Verification items for the finished model (mm, model axes). A direction names the side the tool comes from. Give positions to 0.01 mm unless a question says otherwise; leave off trailing zeros. Loops run counter-clockwise (first coordinate to the right, second up) from the corner with the lowest first, then second, coordinate; pieces in that order, holes last. Notation, with made-up numbers: (68, 18) - (93, 18) arc R11 ccw to (93, 34) - close; hole circle Ø1 at (53, 72.25). An arc over 180 degrees is marked (long way). Use one line per item in the form item = value.
Autodesk Inventor part; units mm, degrees
ref_plane "YZ Plane" through (0, 0, 0) normal (1, 0, 0) x (0, 1, 0)
ref_plane "XZ Plane" through (0, 0, 0) normal (0, 1, 0) x (-1, 0, 0)
ref_plane "XY Plane" through (0, 0, 0) normal (0, 0, 1) x (1, 0, 0)
sketch "Sketch1" plane through (0, 0, 0) normal (0, 0, 1) x (1, 0, 0)
  line L0 (0, 0) -> (0, 125)
  line L1 (0, 125) -> (-105, 10)
  line L2 (-105, 10) -> (-105, 0)
  line L3 (-105, 0) -> (0, 0)
  line L4 (-100, 8.0608) -> (-5, 112.1084)
  line L5 (-5, 112.1084) -> (-5, 5)
  line L6 (-5, 5) -> (-100, 5)
  line L7 (-100, 5) -> (-100, 8.0608)
  point P0 (-52.5, 62.5)
  point P1 (-52.5, 0)
  point P2 (0, 62.5)
  dimension "d0" = 10
  dimension "d1" = 105
  dimension "d2" = 125
  dimension "d3" = 5
extrude "Extrusion1" add sketch "Sketch1" along normal blind 20
sketch "Sketch2" plane through (0, 0, 0) normal (0, 0, -1) x (-1, 0, 0)
  line L0 (5, 112.1084) -> (5, 5)
  line L1 (5, 8.8556) -> (50.4993, 62.2758)
  line L2 (100, 8.0608) -> (5, 112.1084)
  line L3 (5, 5) -> (100, 5)
  line L4 (8.2839, 5) -> (53.8973, 58.5542)
  line L5 (16.4791, 22.3331) -> (16.4791, 99.536)
  line L6 (21.4791, 94.0598) -> (21.4791, 28.2035)
  line L7 (24.1213, 23.5946) -> (85.817, 23.5946)
  line L8 (19.8627, 18.5946) -> (90.3822, 18.5946)
  line L9 (100, 5) -> (100, 8.0608)
  line L10 (100, 6.5304) -> (23.4466, 22.8023)
  line L11 (83.1512, 5) -> (19.7602, 18.4742)
  line L12 (8.1824, 108.6229) -> (21.0073, 27.6496)
  line L13 (5, 96.7537) -> (16.7388, 22.6379)
  point P0 (0, 0)
  point P1 (16.4791, 56.2397)
  point P2 (43.2425, 18.5946)
  point P3 (16.4791, 24.2774)
  dimension "d8" = 2.5
  dimension "d9" = 2.5
  dimension "d10" = 5
  dimension "d11" = 5
  dimension "d16" = 5
  dimension "d17" = 12
  dimension "d18" = 5
  dimension "d19" = 9
extrude "Extrusion2" add sketch "Sketch2" against normal blind 20 contours L2 L12 L5 L13 L0 | L1 L2 L4 L3 L0 | L13 L1 L5 | L5 L12 L1 L13 | L2 L6 L1 L12 L5 | L11 L4 L8 L10 L9 L3 | L4 L10 L8 | L2 L8 L10 L4 L7
fillet "Fillet1" radius 3 18 edges at (-90.3822, 18.5946, 10) (-53.8973, 58.5542, 10) (-85.817, 23.5946, 10) (-24.1213, 23.5946, 10) (-50.4993, 62.2758, 10) (-21.4791, 94.0598, 10) (-16.4791, 99.536, 10) (-21.4791, 28.2035, 10) (0, 0, 10) (-5, 8.8556, 10) (-8.2839, 5, 10) (-105, 0, 10) (-100, 8.0608, 10) (-105, 10, 10) (0, 125, 10) (-19.7602, 18.4742, 10) (-100, 6.5304, 10) (-8.1824, 108.6229, 10)
fillet "Fillet2" radius 1.5 4 edges at (-16.4791, 56.2397, 10) (-43.2425, 18.5946, 10) (-5, 96.7537, 10) (-83.1512, 5, 10)
sketch "Sketch5" plane through (0, 0, 20) normal (0, 0, 1) x (1, 0, 0)
  line L0 (-102, 0) -> (-3, 0)
  line L1 (-85, 0) -> (-85, -20)
  line L2 (-80, 0) -> (-80, -20)
  line L3 (-80, -20) -> (-85, -20)
  line L4 (-10, 0) -> (-10, -20)
  line L5 (-10, -20) -> (-5, -20)
  line L6 (-5, -20) -> (-5, 0)
  line L7 (-105, 8.8365) -> (-105, 3)
  point P0 (0, 0)
  dimension "d35" = 5
  dimension "d36" = 20
  dimension "d37" = 80
  dimension "d38" = 5
  dimension "d52" = 20
extrude "Extrusion3" add sketch "Sketch5" against normal up to surface (20 mm away)
fillet "Fillet3" radius 1.5 4 edges at (-80, -20, 10) (-85, -20, 10) (-10, -20, 10) (-5, -20, 10)
fillet "Fillet4" radius 10 2 edges at (-80, 0, 10) (-10, 0, 10)
sketch "Sketch6" plane through (-10, -18.5, 0) normal (-1, 0, 0) x (0, 0, 1)
  line L0 (0, -1.5) -> (20, -1.5)
  line L1 (0, 0) -> (0, 8.5)
  point P0 (0, 18.5)
  point P1 (10, 8.5)
  dimension "d50" = 10
  dimension "d51" = 10
hole "Hole2" at (-10, -10, 10) direction (1, 0, 0) diameter 5.8 end through all
sketch "Sketch7" plane through (-10, -18.5, 0) normal (-1, 0, 0) x (0, 0, 1)
  arc A0 (12.9, 8.5) -> (7.1, 8.5) centre (10, 8.5) ccw
  circle A1 centre (10, 8.5) radius 6.4
  arc A2 (7.1, 8.5) -> (12.9, 8.5) centre (10, 8.5) ccw
  point P0 (0, 18.5)
  dimension "d53" = 3.5
extrude "Extrusion4" cut sketch "Sketch7" along normal blind 10 contours A2 A0 | A1
sketch "Sketch8" plane through (-80, -18.5, 20) normal (1, 0, 0) x (0, 0, -1)
  line L0 (20, 8.5) -> (20, 0)
  line L1 (0, -1.5) -> (20, -1.5)
  point P0 (20, 18.5)
  point P1 (10, 8.5)
  dimension "d63" = 10
  dimension "d64" = 10
hole "Hole3" at (-80, -10, 10) direction (-1, 0, 0) diameter 5.8 end through all
sketch "Sketch9" plane through (-80, -18.5, 20) normal (1, 0, 0) x (0, 0, -1)
  line L0 (7.1, 8.5) -> (12.9, 8.5)
  circle A0 centre (10, 8.5) radius 6.4
  point P0 (20, 18.5)
extrude "Extrusion5" cut sketch "Sketch9" along normal blind 10
equation "\"d9\" = d8"
equation "\"d35\" = d38"
properties part number "Controls Mid Support"
1. Depth check by flat-ended pin: pin 1 Ø6 at (x, z) = (-43.5, 7) entering from +Y; pin 2 Ø1.6 at (x, z) = (-3.5, 8.5) entering from -Y; pin 3 Ø3 at (x, y) = (-71, 49) entering from +Z; pin 4 Ø10 at (y, z) = (54.5, 7.5) entering from -X. Enter the tip coordinate at first touch or a pass-through.
Result set:
pin_1 = 80.64
pin_2 = 0
pin_3 = 20
pin_4 = -68.93
2. Section check B-B, the plane z = 11. State how many separate pieces and enclosed holes the cut face has, then the cut area to 3 significant figures.
Result set:
separate_pieces = 3
enclosed_holes = 6
area = 3,920 mm²
3. Scan lines: probe 1 along Z at (x, y) = (-6.95, -10); probe 2 along Y at (x, z) = (-6.05, 10); probe 3 along X at (y, z) = (87, 3.5). Record each from-to range of solid material in increasing order.
Result set:
probe_1 = 0 to 7.1, 12.9 to 20
probe_2 = -19.93 to -12.9, -7.1 to 14.72, 79.13 to 118.37
probe_3 = -34.7 to -27.93, -21.56 to -16.48, -11.61 to 0
4. Section check A-A, the plane x = -54. Record the cut outline in (y, z).
Result set:
outline = (0, 0) - (5, 0) - (5, 20) - (0, 20) - close; (11.2, 0) - (23.59, 0) - (23.59, 20) - (11.2, 20) - close; (57.02, 0) - (65.86, 0) - (65.86, 20) - (57.02, 20) - close
5. Tool access check on faces 5 (the cylindrical face through (-79.1, -3.6, 10.1)), 6 (the flat face through (-13.3, 18.6, 9.9)), 7 (the cylindrical face through (-14, -2, 10)). Record the directions out of +Z, -Z, +X, -X, +Y, -Y that give a thin tool (end or side, any length) a straight path to the whole face; none if there is none.
Result set:
face_5 = -Y
face_6 = +Z, -Z
face_7 = +Z, -Z, -Y
6. Draft check along X on faces 1 (the flat face through (-54.022, 65.833, 9.86)), 2 (the flat face through (-94, 0, 10)), 3 (the cylindrical face through (-7.012, 14.172, 10.14)), 4 (the flat face through (-5, -7, 12)). Enter one of: released by +X, released by -X, zero draft, split by the parting line, or undercut.
Result set:
face_1 = released by -X
face_2 = zero draft
face_3 = undercut
face_4 = released by +X
7. Section check D-D, the plane y = 104. Record the cut outline in (x, z).
Result set:
outline = (-19.17, 0) - (0, 0) - (0, 20) - (-19.17, 20) - close
